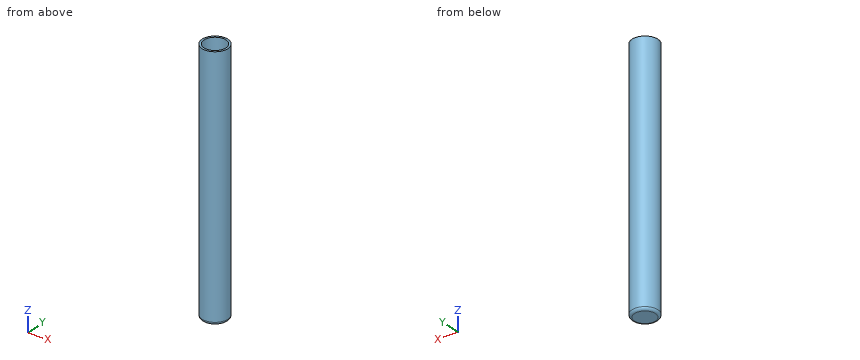
```python
from build123d import *

# Parameters (mm, degrees)
CROQUIS2_R              = 15
SALIENTE_EXTRUIR1_DEPTH = 290
CROQUIS3_R              = 12.7
CORTAR_EXTRUIR1_DEPTH   = 282
REDONDEO1_R             = 3


with BuildPart() as part:
    # Croquis2 → Saliente-Extruir1 (new body)
    with BuildSketch(Plane.XY):
        Circle(CROQUIS2_R)
    extrude(amount=-SALIENTE_EXTRUIR1_DEPTH)

    # Croquis3 → Cortar-Extruir1 (cut)
    with BuildSketch(Plane.XY):
        Circle(CROQUIS3_R)
    extrude(amount=-CORTAR_EXTRUIR1_DEPTH, mode=Mode.SUBTRACT)

    # Redondeo1
    redondeo1_edges = [part.edges().sort_by_distance(p)[0] for p in [
        (-15, 0, -290),
    ]]
    fillet(redondeo1_edges, radius=REDONDEO1_R)


solid = part.part
```
Source: CAD feature listing. Evaluate the final solid. Frame: model axes, mm. Coordinates: 2 decimals unless noted, no trailing zeros. Write each loop counter-clockwise with the first axis right and the second up, starting at its lowest first coordinate (ties: lowest second). Pieces come first, ordered by that corner, then holes. Notation, with made-up numbers: (61, -11) - (88, -11) arc R36 ccw to (88, 25) - close; hole circle Ø7 at (-13, 81.5). An arc over 180 degrees is marked (long way). Answer as a JSON object with one key per item and string values.
Q1. Section query A-A, the plane x = 0. Output: boundary loops of the cut face in (y, z).
Ans:
{"outline": "(-15, -287) arc R3 ccw to (-12, -290) - (12, -290) arc R3 ccw to (15, -287) - (15, 0) - (12.7, 0) - (12.7, -282) - (-12.7, -282) - (-12.7, 0) - (-15, 0) - close"}
Q2. Section query C-C, the plane z = -135. Output: boundary loops of the cut face in (x, y).
Ans:
{"outline": "circle Ø30 at (0, 0); hole circle Ø25.4 at (0, 0)"}
Q3. Material intervals for line 1 (Y direction, x = 0, z = -225); line 2 (X direction, y = 0.5, z = -106); line 3 (Z direction, x = -1.75, y = -5.5), sorted ascending. Write a range as [from, to].
Ans:
{"line 1": "y = [-15, -12.7], [12.7, 15]", "line 2": "x = [-14.99, -12.69], [12.69, 14.99]", "line 3": "z = [-290, -282]"}
Q4. First-contact query: pin 1 Ø6 at (x, z) = (3.5, -158.5) entering from +Y; pin 2 Ø6 at (x, y) = (2.5, -1) entering from +Z; pin 3 Ø1.5 at (x, z) = (2.5, -197) entering from +Y. Flat tips, straight axial feed; report the tip coordinate or a pass-through.
Ans:
{"pin 1": "stops at y = 14.99", "pin 2": "stops at z = -282", "pin 3": "stops at y = 14.9"}
